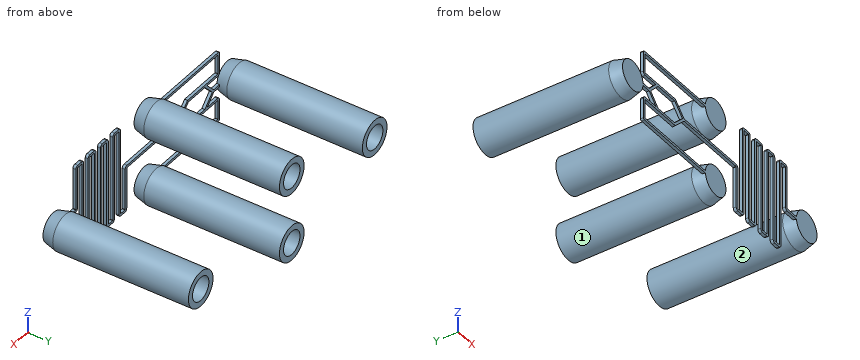
from build123d import *

# Parameters (mm, degrees)
SKELTON_EXTRU_DEPTH = 1
SKETCH8_R           = 4
CUT_EXTRUDE1_DEPTH  = 45


with BuildPart() as part:
    # Sketch2 → skelton_extru (new body)
    with BuildSketch(Plane(origin=(0, 0, 0), x_dir=(1, 0, 0), z_dir=(0, 1, 0))):
        with BuildLine():
            Line((-31.842640687, 11.242640687), (2.6, 11.242640687))
            ThreePointArc((2.6, 11.242640687), (3, 11.642640687), (2.6, 12.042640687))
            Line((2.6, 12.042640687), (-31.842640687, 12.042640687))
            Line((-31.842640687, 12.042640687), (-32.142640687, 12.042640687))
            ThreePointArc((-32.142640687, 12.042640687), (-32.496194078, 11.896194078), (-32.642640687, 11.542640687))
            Line((-32.642640687, 11.542640687), (-32.642640687, 4.742640687))
            ThreePointArc((-32.642640687, 4.742640687), (-32.37903679, 4.106244584), (-31.742640687, 3.842640687))
            Line((-31.742640687, 3.842640687), (-26.585761453, 3.842640687))
            Line((-26.585761453, 3.842640687), (-29.831514219, 0.4))
            Line((-29.831514219, 0.4), (-37.831514219, 0.4))
            ThreePointArc((-37.831514219, 0.4), (-38.231514219, 0), (-37.831514219, -0.4))
            Line((-37.831514219, -0.4), (-29.831514219, -0.4))
            Line((-29.831514219, -0.4), (-26.585761453, -3.842640687))
            Line((-26.585761453, -3.842640687), (-31.742640687, -3.842640687))
            ThreePointArc((-31.742640687, -3.842640687), (-32.37903679, -4.106244584), (-32.642640687, -4.742640687))
            Line((-32.642640687, -4.742640687), (-32.642640687, -11.542640687))
            ThreePointArc((-32.642640687, -11.542640687), (-32.496194078, -11.896194078), (-32.142640687, -12.042640687))
            Line((-32.142640687, -12.042640687), (-31.842640687, -12.042640687))
            Line((-31.842640687, -12.042640687), (2.6, -12.042640687))
            ThreePointArc((2.6, -12.042640687), (3, -11.642640687), (2.6, -11.242640687))
            Line((2.6, -11.242640687), (-31.842640687, -11.242640687))
            Line((-31.842640687, -11.242640687), (-31.842640687, -4.742640687))
            ThreePointArc((-31.842640687, -4.742640687), (-31.813351365, -4.671930009), (-31.742640687, -4.642640687))
            Line((-31.742640687, -4.642640687), (-17.076955262, -4.642640687))
            Line((-17.076955262, -4.642640687), (-12.834314575, -0.4))
            Line((-12.834314575, -0.4), (6.7, -0.4))
            Line((6.7, -0.4), (12.5, -0.4))
            ThreePointArc((12.5, -0.4), (13.136396103, -0.136396103), (13.4, 0.5))
            Line((13.4, 0.5), (13.4, 14.5))
            ThreePointArc((13.4, 14.5), (13.429289322, 14.570710678), (13.5, 14.6))
            Line((13.5, 14.6), (15.5, 14.6))
            ThreePointArc((15.5, 14.6), (15.570710678, 14.570710678), (15.6, 14.5))
            Line((15.6, 14.5), (15.6, 0))
            Line((15.6, 0), (15.6, -14.5))
            ThreePointArc((15.6, -14.5), (15.863603897, -15.136396103), (16.5, -15.4))
            Line((16.5, -15.4), (18.5, -15.4))
            ThreePointArc((18.5, -15.4), (19.136396103, -15.136396103), (19.4, -14.5))
            Line((19.4, -14.5), (19.4, 14.5))
            ThreePointArc((19.4, 14.5), (19.429289322, 14.570710678), (19.5, 14.6))
            Line((19.5, 14.6), (21.5, 14.6))
            ThreePointArc((21.5, 14.6), (21.570710678, 14.570710678), (21.6, 14.5))
            Line((21.6, 14.5), (21.6, -14.5))
            ThreePointArc((21.6, -14.5), (21.863603897, -15.136396103), (22.5, -15.4))
            Line((22.5, -15.4), (24.5, -15.4))
            ThreePointArc((24.5, -15.4), (25.136396103, -15.136396103), (25.4, -14.5))
            Line((25.4, -14.5), (25.4, 14.5))
            ThreePointArc((25.4, 14.5), (25.429289322, 14.570710678), (25.5, 14.6))
            Line((25.5, 14.6), (27.5, 14.6))
            ThreePointArc((27.5, 14.6), (27.570710678, 14.570710678), (27.6, 14.5))
            Line((27.6, 14.5), (27.6, -14.5))
            ThreePointArc((27.6, -14.5), (27.863603897, -15.136396103), (28.5, -15.4))
            Line((28.5, -15.4), (30.5, -15.4))
            ThreePointArc((30.5, -15.4), (31.136396103, -15.136396103), (31.4, -14.5))
            Line((31.4, -14.5), (31.4, 14.5))
            ThreePointArc((31.4, 14.5), (31.429289322, 14.570710678), (31.5, 14.6))
            Line((31.5, 14.6), (33.5, 14.6))
            ThreePointArc((33.5, 14.6), (33.570710678, 14.570710678), (33.6, 14.5))
            Line((33.6, 14.5), (33.6, -14.5))
            ThreePointArc((33.6, -14.5), (33.863603897, -15.136396103), (34.5, -15.4))
            Line((34.5, -15.4), (36.5, -15.4))
            ThreePointArc((36.5, -15.4), (37.136396103, -15.136396103), (37.4, -14.5))
            Line((37.4, -14.5), (37.4, -0.5))
            ThreePointArc((37.4, -0.5), (37.429289322, -0.429289322), (37.5, -0.4))
            Line((37.5, -0.4), (47, -0.4))
            ThreePointArc((47, -0.4), (47.4, 0), (47, 0.4))
            Line((47, 0.4), (37.5, 0.4))
            ThreePointArc((37.5, 0.4), (36.863603897, 0.136396103), (36.6, -0.5))
            Line((36.6, -0.5), (36.6, -14.5))
            ThreePointArc((36.6, -14.5), (36.570710678, -14.570710678), (36.5, -14.6))
            Line((36.5, -14.6), (34.5, -14.6))
            ThreePointArc((34.5, -14.6), (34.429289322, -14.570710678), (34.4, -14.5))
            Line((34.4, -14.5), (34.4, 14.5))
            ThreePointArc((34.4, 14.5), (34.136396103, 15.136396103), (33.5, 15.4))
            Line((33.5, 15.4), (31.5, 15.4))
            ThreePointArc((31.5, 15.4), (30.863603897, 15.136396103), (30.6, 14.5))
            Line((30.6, 14.5), (30.6, -14.5))
            ThreePointArc((30.6, -14.5), (30.570710678, -14.570710678), (30.5, -14.6))
            Line((30.5, -14.6), (28.5, -14.6))
            ThreePointArc((28.5, -14.6), (28.429289322, -14.570710678), (28.4, -14.5))
            Line((28.4, -14.5), (28.4, 14.5))
            ThreePointArc((28.4, 14.5), (28.136396103, 15.136396103), (27.5, 15.4))
            Line((27.5, 15.4), (25.5, 15.4))
            ThreePointArc((25.5, 15.4), (24.863603897, 15.136396103), (24.6, 14.5))
            Line((24.6, 14.5), (24.6, -14.5))
            ThreePointArc((24.6, -14.5), (24.570710678, -14.570710678), (24.5, -14.6))
            Line((24.5, -14.6), (22.5, -14.6))
            ThreePointArc((22.5, -14.6), (22.429289322, -14.570710678), (22.4, -14.5))
            Line((22.4, -14.5), (22.4, 14.5))
            ThreePointArc((22.4, 14.5), (22.136396103, 15.136396103), (21.5, 15.4))
            Line((21.5, 15.4), (19.5, 15.4))
            ThreePointArc((19.5, 15.4), (18.863603897, 15.136396103), (18.6, 14.5))
            Line((18.6, 14.5), (18.6, -14.5))
            ThreePointArc((18.6, -14.5), (18.570710678, -14.570710678), (18.5, -14.6))
            Line((18.5, -14.6), (16.5, -14.6))
            ThreePointArc((16.5, -14.6), (16.429289322, -14.570710678), (16.4, -14.5))
            Line((16.4, -14.5), (16.4, 0))
            Line((16.4, 0), (16.4, 14.5))
            ThreePointArc((16.4, 14.5), (16.136396103, 15.136396103), (15.5, 15.4))
            Line((15.5, 15.4), (13.5, 15.4))
            ThreePointArc((13.5, 15.4), (12.863603897, 15.136396103), (12.6, 14.5))
            Line((12.6, 14.5), (12.6, 0.5))
            ThreePointArc((12.6, 0.5), (12.570710678, 0.429289322), (12.5, 0.4))
            Line((12.5, 0.4), (6.7, 0.4))
            Line((6.7, 0.4), (-12.834314575, 0.4))
            Line((-12.834314575, 0.4), (-17.076955262, 4.642640687))
            Line((-17.076955262, 4.642640687), (-31.742640687, 4.642640687))
            ThreePointArc((-31.742640687, 4.642640687), (-31.813351365, 4.671930009), (-31.842640687, 4.742640687))
            Line((-31.842640687, 4.742640687), (-31.842640687, 11.242640687))
        make_face()
        Polygon((-13.565685425, 0), (-17.408326112, -3.842640687), (-25.486266619, -3.842640687), (-29.109143003, 0), (-25.486266619, 3.842640687), (-17.408326112, 3.842640687), align=None, mode=Mode.SUBTRACT)
    extrude(amount=SKELTON_EXTRU_DEPTH)

    # Sketch3 → Revolve1 (revolve)
    with BuildSketch(Plane.XY.offset(-11.642640687), mode=Mode.PRIVATE) as revolve1_sk:
        Polygon((2.6, 0), (7.6, 0), (8.6, 4), (8.6, 50), (2.6, 50), align=None)
    revolve(revolve1_sk.sketch.rotate(Axis((2.6, 0, -11.642640687), (0, 1, 0)), 184.588565502), axis=Axis((2.6, 0, -11.642640687), (0, 1, 0)))

    # Sketch4 → Revolve2 (revolve)
    with BuildSketch(Plane(origin=(0, 0, 0), x_dir=(-1, 0, 0), z_dir=(0, 0, -1)), mode=Mode.PRIVATE) as revolve2_sk:
        Polygon((-47, 0), (-52, 0), (-53, 4), (-53, 50), (-47, 50), align=None)
    revolve(revolve2_sk.sketch.rotate(Axis((47, 0, 0), (0, 1, 0)), 184.588558424), axis=Axis((47, 0, 0), (0, 1, 0)))

    # Sketch5 → Revolve3 (revolve)
    with BuildSketch(Plane(origin=(0, 0, 0), x_dir=(-1, 0, 0), z_dir=(0, 0, -1))):
        Polygon((37.831514219, 50), (37.831514219, 0), (42.831514219, 0), (43.831514219, 4), (43.831514219, 50), align=None)
    revolve(axis=Axis((-37.831514219, 50, 0), (0, -1, 0)))

    # Sketch6 → Revolve4 (revolve)
    with BuildSketch(Plane.XY.offset(11.642640687), mode=Mode.PRIVATE) as revolve4_sk:
        Polygon((2.6, 0), (7.6, 0), (8.6, 4), (8.6, 50), (2.6, 50), align=None)
    revolve(revolve4_sk.sketch.rotate(Axis((2.6, 0, 11.642640687), (0, 1, 0)), 184.588565502), axis=Axis((2.6, 0, 11.642640687), (0, 1, 0)))

    # Sketch8 → Cut-Extrude1 (cut)
    with BuildSketch(Plane(origin=(0, 50, 0), x_dir=(1, 0, 0), z_dir=(0, 1, 0))):
        with Locations(Location((-37.831514219, 0, 0), (0, 0, 180))):
            Circle(SKETCH8_R)
        with Locations(Location((2.6, 11.642640687, 0), (0, 0, 180))):
            Circle(SKETCH8_R)
        with Locations(Location((2.6, -11.642640687, 0), (0, 0, 180))):
            Circle(SKETCH8_R)
        with Locations(Location((47, 0, 0), (0, 0, 180))):
            Circle(SKETCH8_R)
    extrude(amount=-CUT_EXTRUDE1_DEPTH, mode=Mode.SUBTRACT)


solid = part.part
Could you check a few things on this model? Use its own coordinates, in mm. Face numbers are marked on the shaded views. Round coordinates to 2 decimals unless told otherwise and drop trailing zeros. Write each loop counter-clockwise with the first axis right and the second up, starting at its lowest first coordinate (ties: lowest second). Pieces come first, ordered by that corner, then holes. Notation, with made-up numbers: (-1.5, -8.5) - (18.5, -8.5) arc R11 ccw to (18.5, 5.5) - close; hole circle Ø3 at (-23, 12.25). An arc over 180 degrees is marked (long way). Put each result on its own line as item: value. Start each with the question number.
(1) Thinking about a two-plate mould opening in Z: for the marked faces 1 and 2, which applies, released by +Z, released by -Z, zero draft, split by the parting line, or undercut?
(2) Will these pins go through, and if not, where does the flat tip stop? pin 1 (1.1 mm diameter, centred on x = 26.5, y = 0.5, fed in from +Z); pin 2 (1.1 mm diameter, centred on y = 0.5, z = 9, fed in from +X); pin 3 (0.5 mm diameter, centred on y = 0.5, z = 4, fed in from +X); pin 4 (10 mm diameter, centred on x = -11, y = 20.5, fed in from +Z).
(3) I want a section at A-A, the plane y = 35.5. Please give me the cut outline in (x, z).
(4) I want a section at C-C, the plane x = 2.6. Please give me the cut outline in (y, z), plus the area to 3 significant figures.
(5) I need wall thicknesses on probe 1 along Z at (x, y) = (2.6, 39); probe 2 along Z at (x, y) = (2, 15); probe 3 along Z at (x, y) = (47, 14). Which ranges of each line are inside material? Lowest first, please.
(6) I want a section at B-B, the plane x = 47. Please give me the cut outline in (y, z), plus the area to 3 significant figures.
Here are the results:
1. face 1: undercut
1. face 2: split by the parting line
2. pin 1: stops at z = -14.6
2. pin 2: stops at x = 37.4
2. pin 3: stops at x = 50.51
2. pin 4: passes through
3. outline: circle Ø12 at (-37.83, 0); circle Ø12 at (2.6, -11.64); circle Ø12 at (2.6, 11.64); circle Ø12 at (47, 0); hole circle Ø8 at (-37.83, 0); hole circle Ø8 at (2.6, -11.64); hole circle Ø8 at (2.6, 11.64); hole circle Ø8 at (47, 0)
4. outline: (0, -16.64) - (4, -17.64) - (50, -17.64) - (50, -15.64) - (5, -15.64) - (5, -7.64) - (50, -7.64) - (50, -5.64) - (4, -5.64) - (0, -6.64) - close; (0, -0.4) - (1, -0.4) - (1, 0.4) - (0, 0.4) - close; (0, 6.64) - (4, 5.64) - (50, 5.64) - (50, 7.64) - (5, 7.64) - (5, 15.64) - (50, 15.64) - (50, 17.64) - (4, 17.64) - (0, 16.64) - close
4. area: 473 mm^2
5. probe 1: z = -17.64 to -15.64, -7.64 to -5.64, 5.64 to 7.64, 15.64 to 17.64
5. probe 2: z = -17.61 to -15.6, -7.69 to -5.67, 5.67 to 7.69, 15.6 to 17.61
5. probe 3: z = -6 to -4, 4 to 6
6. outline: (0, -5) - (4, -6) - (50, -6) - (50, -4) - (5, -4) - (5, 4) - (50, 4) - (50, 6) - (4, 6) - (0, 5) - close
6. area: 236 mm^2
